Geometry check sheet. Reference: the model listing, model coordinates, mm. A direction names the side the tool comes from. Coordinates: 2 decimals unless noted, no trailing zeros. Loops run counter-clockwise (first coordinate to the right, second up) from the corner with the lowest first, then second, coordinate; pieces in that order, holes last.
Autodesk Inventor part; units mm, degrees
ref_plane "YZ Plane" through (0, 0, 0) normal (1, 0, 0) x (0, 1, 0)
ref_plane "XZ Plane" through (0, 0, 0) normal (0, 1, 0) x (-1, 0, 0)
ref_plane "XY Plane" through (0, 0, 0) normal (0, 0, 1) x (1, 0, 0)
sketch "Sketch1" plane through (0, 0, 0) normal (0, 1, 0) x (-1, 0, 0)
  circle A0 centre (0, 0) radius 12
  circle A1 centre (0, 0) radius 22.5
  line L0 (11.619, 3) -> (16.619, 3)
  line L1 (16.619, 3) -> (16.619, -3)
  line L2 (16.619, -3) -> (11.619, -3)
  line L3 (11.619, -3) -> (11.619, 3)
  dimension "d0" = 24
  dimension "d1" = 45
  dimension "d2" = 6
  dimension "d3" = 5
extrude "Extrusion1" add sketch "Sketch1" along normal blind 40
sketch "Sketch2" plane through (0, 40, 0) normal (0, 1, 0) x (1, 0, 0)
  circle A0 centre (0, 0) radius 22.5
extrude "Extrusion2" add sketch "Sketch2" along normal blind 8
sketch "Sketch3" plane through (0, 48, 0) normal (0, 1, 0) x (1, 0, 0)
  circle A0 centre (0, 0) radius 12
  dimension "d29" = 24
extrude "Extrusion3" add sketch "Sketch3" along normal blind 25
sketch "Sketch4" plane through (0, 0, 0) normal (1, 0, 0) x (0, 1, 0)
  circle A0 centre (63, 0) radius 1.75
  line L0 (48, -22.5) -> (48, 22.5)
  point P0 (0, 0)
  dimension "d10" = 15
  dimension "d11" = 3.5
extrude "Extrusion4" cut sketch "Sketch4" along normal through all both and the other way through all
sketch "Sketch5" plane through (0, 0, 0) normal (0, 0, 1) x (1, 0, 0)
  circle A0 centre (0, 63) radius 1.75
  line L0 (-12, 64.75) -> (12, 64.75)
  line L1 (22.5, 48) -> (-22.5, 48)
  point P0 (0, 0)
  dimension "d14" = 15
extrude "Extrusion5" cut sketch "Sketch5" along normal through all both and the other way through all
sketch "Sketch6" plane through (0, 0, 0) normal (1, 0, 0) x (0, 1, 0)
  circle A0 centre (24, 0) radius 2
  line L0 (0, -22.5) -> (0, 22.5)
  line L1 (48, -22.5) -> (48, 22.5)
  point P0 (0, 0)
  dimension "d18" = 4
  dimension "d19" = 24
  dimension "d20" = 24
extrude "Extrusion6" cut sketch "Sketch6" along normal through all
chamfer "Chamfer1" distance 3 angle 45 1 edges at (-22.5, 48, 0)
chamfer "Chamfer2" distance 5 angle 45 1 edges at (-12, 48, 0)
equation "\"d19\" = d20"
properties part number "shaft adapter"
1) Section check A-A on y = 63. Record the cut outline in (x, z), and give its area (3 significant figures).
Data:
outline: (-11.87, -1.75) arc R12 ccw to (-1.75, -11.87) - (-1.75, -1.75) - close; (-11.87, 1.75) - (-1.75, 1.75) - (-1.75, 11.87) arc R12 ccw to start; (1.75, -11.87) arc R12 ccw to (11.87, -1.75) - (1.75, -1.75) - close; (1.75, 1.75) - (11.87, 1.75) arc R12 ccw to (1.75, 11.87) - close
area: 297 mm2
2) Depth check by flat-ended pin: pin 1 (5 mm diameter, centred on x = -17, y = 34.5, fed in from +Z); pin 2 (19 mm diameter, centred on x = -9, z = 3.5, fed in from -Y); pin 3 (4 mm diameter, centred on x = 0, y = 63, fed in from +Z); pin 4 (2.5 mm diameter, centred on x = -14, y = 21.5, fed in from +Z). Enter the tip coordinate at first touch or a pass-through.
Data:
pin 1: stops at z = 17.2
pin 2: stops at y = 0
pin 3: stops at z = 12
pin 4: stops at z = 18.54
3) Access from +Z, -Z, +X, -X, +Y, -Y to the whole of each face (thin tool, end or side, straight path). Record for faces 1 (the flat face through (-14, 20, 3)), 2 (the cylindrical face through (11.085, 62.86, -4.596)), 3 (the cylindrical face through (-5.916, 62.772, 1.735)).
Data:
face 1: -Y
face 2: +Y
face 3: +X, -X
4) Section check B-B on y = 46. Record the cut outline in (x, z).
Data:
outline: circle Ø43 at (0, 0)
5) Material ranges on probe 1 along Y at (x, z) = (-9.5, 0); probe 2 along Z at (x, y) = (-0.5, 36.5); probe 3 along X at (y, z) = (12, 0), recorded low to high.
Data:
probe 1: y = 40 to 61.25, 64.75 to 73
probe 2: z = -22.49 to -11.99, 11.99 to 22.49
probe 3: x = -22.5 to -16.62, 12 to 22.5
6) Section check C-C on y = 19. Record the cut outline in (x, z).
Data:
outline: circle Ø45 at (0, 0); hole (-16.62, -3) - (-11.62, -3) arc R12 ccw (long way) to (-11.62, 3) - (-16.62, 3) - close
7) Mould release check, pull along Y, two halves, no side actions. Record for faces 4 (the cylindrical face through (17, 22, 0)), 5 (the conical face through (5.7, 52.7, -10.9)), 6 (the flat face through (-14, 20, -3)): +Y half, -Y half, draft (parallel to the pull), parting line (faces both ways), or undercut.
Data:
face 4: undercut
face 5: +Y half
face 6: draft
